Input: part model. Units: mm. Frame: model coordinates. Coordinates: 2 decimals unless noted, no trailing zeros. Write each loop counter-clockwise with the first axis right and the second up, starting at its lowest first coordinate (ties: lowest second). Pieces come first, ordered by that corner, then holes. Notation, with made-up numbers: M 16,-27 L 49,-27 A33 cw 49,1 Z; hole C 2,28 d1. An arc over 180 degrees is marked long. Use one line per item in the form item = value.
from build123d import *

# Parameters (mm, degrees)
BOSS_EXTRUDE1_DEPTH = 3.175
BOSS_EXTRUDE2_DEPTH = 3.175


with BuildPart() as part:
    # Sketch1 → Boss-Extrude1 (new body)
    with BuildSketch(Plane.XY):
        Polygon((0, 143.6878), (25.4, 143.6878), (25.4, 146.8628), (50.8, 146.8628), (50.8, 143.6878), (152.4, 143.6878), (152.4, 146.8628), (177.8, 146.8628), (177.8, 143.6878), (203.2, 143.6878), (203.2, 0), (0, 0), align=None)
    extrude(amount=BOSS_EXTRUDE1_DEPTH)

    # Sketch1<2> → Boss-Extrude2 (add)
    with BuildSketch(Plane.XY):
        Polygon((0, 143.6878), (25.4, 143.6878), (25.4, 146.8628), (50.8, 146.8628), (50.8, 143.6878), (152.4, 143.6878), (152.4, 146.8628), (177.8, 146.8628), (177.8, 143.6878), (203.2, 143.6878), (203.2, 0), (0, 0), align=None)
    extrude(amount=BOSS_EXTRUDE2_DEPTH)


solid = part.part
(1) First-contact query: pin 1 Ø1.6 at (x, z) = (194, 2) entering from +Y; pin 2 Ø1.6 at (y, z) = (145, 2.5) entering from +X. Flat tips, straight axial feed; report the tip coordinate or a pass-through.
Computed:
pin_1 = 143.69
pin_2 = 177.8
(2) Section query A-A on z = 1.3. Return the cut outline in (x, y).
Computed:
outline = M 0,0 L 203.2,0 L 203.2,143.69 L 177.8,143.69 L 177.8,146.86 L 152.4,146.86 L 152.4,143.69 L 50.8,143.69 L 50.8,146.86 L 25.4,146.86 L 25.4,143.69 L 0,143.69 Z
(3) Section query B-B on x = 92.5. Return the cut outline in (y, z) (3 decimals), plus the area to 3 significant figures.
Computed:
outline = M 0,0 L 143.688,0 L 143.688,3.175 L 0,3.175 Z
area = 456 mm^2
(4) Line query: probe 1 along Y at (x, z) = (22, 2). Output: solid intervals per line, ascending.
Computed:
probe_1 = 0 to 143.69
